Input: part model. Units: mm. Frame: model coordinates. Face numbers are marked on the shaded views. A direction names the side the tool comes from. Round coordinates to 2 decimals unless told otherwise and drop trailing zeros. Order: outer loops, then holes, each group sorted by start corner. A loop starts at its lowest first (then second) coordinate and runs counter-clockwise, first axis right, second up. Notation, with made-up numbers: M 27,46 L 33,46 A16 cw 33,67 Z; hole C -26,52 d9. An arc over 180 degrees is marked long. One line per question, with ' | ' between items.
Autodesk Inventor part; units mm, degrees
ref_plane "YZ Plane" through (0, 0, 0) normal (1, 0, 0) x (0, 1, 0)
ref_plane "XZ Plane" through (0, 0, 0) normal (0, 1, 0) x (-1, 0, 0)
ref_plane "XY Plane" through (0, 0, 0) normal (0, 0, 1) x (1, 0, 0)
sketch "Sketch1" plane through (0, 0, 0) normal (0, 1, 0) x (-1, 0, 0)
  line L0 (41.275, 41.275) -> (-41.275, 41.275)
  line L1 (-41.275, 41.275) -> (-41.275, -41.275)
  line L2 (-41.275, -41.275) -> (41.275, -41.275)
  line L3 (41.275, -41.275) -> (41.275, 41.275)
  circle A0 centre (0, 0) radius 44.45 construction
  circle A1 centre (0, 0) radius 39.6875
  line L4 (-41.275, 41.275) -> (41.275, -41.275) construction
  line L5 (41.275, 41.275) -> (-41.275, -41.275) construction
  circle A2 centre (31.4309, 31.4309) radius 2.159
  circle A3 centre (31.4309, -31.4309) radius 2.159
  circle A4 centre (-31.4309, 31.4309) radius 2.159
  circle A5 centre (-31.4309, -31.4309) radius 2.159
  point P0 (0, 0)
  point P1 (0, 0)
  point P2 (0, 0)
  dimension "d0" = 82.55
  dimension "d1" = 82.55
  dimension "d2" = 88.9
  dimension "d3" = 79.375
  dimension "d4" = 4.318
  dimension "d5" = 4.318
  dimension "d6" = 4.318
  dimension "d7" = 4.318
extrude "Extrusion1" add sketch "Sketch1" along normal blind 3.175 contours L3 L2 L1 L0 | A1
sketch "Sketch2" plane through (0, 3.175, 0) normal (0, 1, 0) x (1, 0, 0)
  circle A0 centre (0, 0) radius 39.0525
  circle A1 centre (0, 0) radius 39.6875 construction
  point P0 (0, 0)
  dimension "d10" = 78.105
  dimension "d17" = 79.375
extrude "Extrusion2" add sketch "Sketch2" along normal blind 1.905
fillet "Fillet1" radius 3.175 1 edges at (41.275, 1.5875, 41.275)
fillet "Fillet2" radius 3.175 1 edges at (-41.275, 1.5875, 41.275)
fillet "Fillet3" radius 3.175 1 edges at (41.275, 1.5875, -41.275)
fillet "Fillet4" radius 3.175 1 edges at (-41.275, 1.5875, -41.275)
properties part number "3-125-instrument-blank"
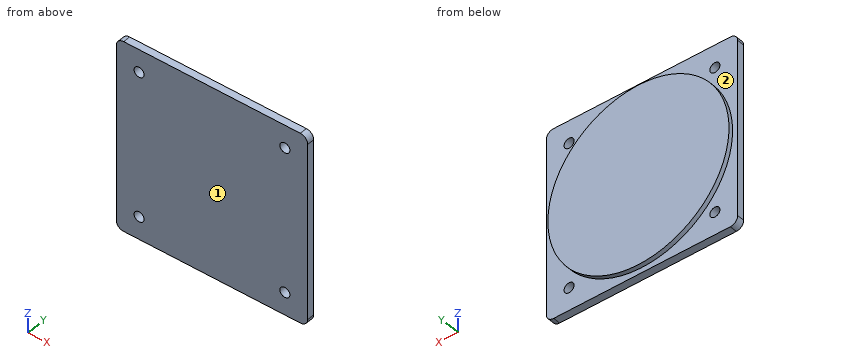
Item 1: Section query B-B, the plane x = 0. Return loops of the section in (y, z) (1 decimal), plus the area to 3 significant figures.
Report:
outline: M 0,-41.3 L 3.2,-41.3 L 3.2,-39.1 L 5.1,-39.1 L 5.1,39.1 L 3.2,39.1 L 3.2,41.3 L 0,41.3 Z | area: 411 mm²
Item 2: Section query C-C, the plane z = 32.5. Return loops of the section in (x, y) (3 decimals), plus the area to 3 significant figures.
Report:
outline: M -41.275,0 L -33.307,0 L -33.307,3.175 L -41.275,3.175 Z; M -29.555,0 L 29.555,0 L 29.555,3.175 L 21.653,3.175 L 21.653,5.08 L -21.653,5.08 L -21.653,3.175 L -29.555,3.175 Z; M 33.307,0 L 41.275,0 L 41.275,3.175 L 33.307,3.175 Z | area: 321 mm²
Item 3: Line query: line 1 along Z through (x, y) = (31.5, 2) (3 decimals); line 2 along Z through (x, y) = (29.5, 2) (3 decimals); line 3 along X through (y, z) = (0.8, 30.5) (3 decimals). Output: solid intervals per line, ascending. Write a range as from..to.
Report:
line 1: -41.275..-33.589, -29.273..29.273, 33.589..41.275 | line 2: -41.275..-32.397, -30.465..30.465, 32.397..41.275 | line 3: -41.275..-33.379, -29.483..29.483, 33.379..41.275
Item 4: Access query for the marked faces 1 and 2. Directions: +Z, -Z, +X, -X, +Y, -Y. A direction counts if a zero-diameter tool reaches every point of the face in a straight line with its end or side. Return the directions, or none.
Report:
face 1: +Z, -Z, +X, -X, -Y | face 2: +Y
Item 5: Section query A-A, the plane z = 0. Return loops of the section in (x, y) (1 decimal), plus the area to 3 significant figures.
Report:
outline: M -41.3,0 L 41.3,0 L 41.3,3.2 L 39.1,3.2 L 39.1,5.1 L -39.1,5.1 L -39.1,3.2 L -41.3,3.2 Z | area: 411 mm²
Item 6: First-contact query: pin 1 (5 mm diameter, centred on x = -13, z = 26.5, fed in from -Y). Flat tip, straight axial feed; report the tip coordinate or a pass-through.
Report:
pin 1: y = 0
